```python
from build123d import *

# Parameters (mm, degrees)
F3_W     = 135
F3_H     = 135
F4_DEPTH = 20
F0_W     = 15.1
F0_H     = 14.1
F6_START = 14
F6_DEPTH = 136
F7_START = 19
F7_DEPTH = 6


with BuildPart() as f4:
    # F3 (on Top) → F4 (new body)
    with BuildSketch(Plane.XY):
        Rectangle(F3_W, F3_H)
    extrude(amount=F4_DEPTH)

    # F0 (on Front) → F5 (revolve, cut)
    with BuildSketch(Plane.XZ):
        with Locations((7.55, 12.95)):
            Rectangle(F0_W, F0_H)
    revolve(axis=Axis((0, 0, 12.95), (0, 0, -1)), mode=Mode.SUBTRACT)

    # F1 (on Right) → F6 (cut)
    with BuildSketch(Plane.YZ.offset(F6_START)):
        with BuildLine():
            Line((4.5, 20.4638522118), (0, 20.4638522118))
            Line((0, 20.4638522118), (-4.5, 20.4638522118))
            Line((-4.5, 20.4638522118), (-4.5, 10.4638522118))
            ThreePointArc((-4.5, 10.4638522118), (0, 5.9638522118), (4.5, 10.4638522118))
            Line((4.5, 10.4638522118), (4.5, 20.4638522118))
        make_face()
    extrude(amount=F6_DEPTH, mode=Mode.SUBTRACT)

    # F2 (on Top) → F7 (cut)
    with BuildSketch(Plane.XY.offset(F7_START)):
        Polygon((14, 0.5), (14, 0), (14, -0.5), (74, -0.5), (74, 0.5), align=None)
        Polygon((0.5, -14), (0, -14), (-0.5, -14), (-0.5, -74), (0.5, -74), align=None)
        Polygon((-13.9910685796, -0.5), (-13.9910685796, 0), (-13.9910685796, 0.5), (-73.9910685796, 0.5), (-73.9910685796, -0.5), align=None)
        Polygon((-0.5, 73.9972595498), (-0.5, 13.9972595498), (0, 13.9972595498), (0.5, 13.9972595498), (0.5, 73.9972595498), align=None)
    extrude(amount=F7_DEPTH, mode=Mode.SUBTRACT)


solid = f4.part
```
Input: part model. Units: mm. Frame: model coordinates. A direction names the side the tool comes from. Round coordinates to 2 decimals unless told otherwise and drop trailing zeros. Write each loop counter-clockwise with the first axis right and the second up, starting at its lowest first coordinate (ties: lowest second). Pieces come first, ordered by that corner, then holes. Notation, with made-up numbers: (37, 28) -> (45, 28) arc R21 cw to (45, 55) -> close; hole circle Ø8 at (30.25, 37.25). An arc over 180 degrees is marked (long way). Answer as CSV lines item,"result".
1. Mould query, pull axis Y, two halves, no side actions, for faces 4 (the cylindrical face through (-3.27, 14.74, 13.05)), 5 (the flat face through (34, 36, 20)), 6 (the flat face through (-1, -67.5, 10)). Classes: +Y half, -Y half, draft (parallel to the pull), parting line (faces both ways), or undercut.
Geometry says:
face 4,"undercut"
face 5,"draft"
face 6,"-Y half"
2. Reachability of faces 1 (the flat face through (34, -36, 20)), 2 (the flat face through (41, 4.5, 15)), 3 (the flat face through (0, 0, 5.9)) from +Z, -Z, +X, -X, +Y, -Y: full face, straight path, thin tool, end or side. Return the list, or none.
Geometry says:
face 1,"+Z, +X, -X, +Y, -Y"
face 2,"+Z, +X"
face 3,"+Z"
3. Section B-B (z = 16). Return the cut outline in (x, y).
Geometry says:
outline,"(-67.5, -67.5) -> (67.5, -67.5) -> (67.5, -4.5) -> (14.41, -4.5) arc R15.1 cw (long way) to (14.41, 4.5) -> (67.5, 4.5) -> (67.5, 67.5) -> (-67.5, 67.5) -> close"
4. Contact query for flat-ended pins moving along their axis: P1, Ø0.5, axis at x = -35, y = 0, coming from the +Z side; P2, Ø15, axis at x = 0.5, y = 6, coming from the +Z side. Output: stop coordinate, or through.
Geometry says:
P1,"stops at z = 19"
P2,"stops at z = 5.9"
5. Section A-A (x = 43). Return the cut outline in (y, z).
Geometry says:
outline,"(-67.5, 0) -> (67.5, 0) -> (67.5, 20) -> (4.5, 20) -> (4.5, 10.46) arc R4.5 cw to (-4.5, 10.46) -> (-4.5, 20) -> (-67.5, 20) -> close"
6. Ray query, L1, parallel to Y at x = 0, z = 12.5; L2, parallel to Y at x = 49.5, z = 14.75; L3, parallel to Z at x = -39.5, y = 0. Return the intervals inside material, ascending. Write a range as [from, to].
Geometry says:
L1,"y = [-67.5, -15.1], [15.1, 67.5]"
L2,"y = [-67.5, -4.5], [4.5, 67.5]"
L3,"z = [0, 19]"
